The listing builds one solid part. Answer for the finished solid, in the listing's coordinates (mm). Face numbers are marked on the shaded views. A direction names the side the tool comes from. Coordinates: 2 decimals unless noted, no trailing zeros. Write each loop counter-clockwise with the first axis right and the second up, starting at its lowest first coordinate (ties: lowest second). Pieces come first, ordered by that corner, then holes. Notation, with made-up numbers: M -22,-9 L 18,-9 A25 ccw 18,6 Z; hole C -9,20 d5. An arc over 180 degrees is marked long. Put each result on its own line as item: value. Start each with the question number.
```python
from build123d import *

# Parameters (mm, degrees)
F1_DEPTH = 3.68
F2_T     = -1
F3_SIZE2 = 0.5
F3_SIZE  = 1.5
F4_SIZE  = 0.2


with BuildPart() as f1:
    # F0 (on Top) → F1 (new body)
    with BuildSketch(Plane.XY):
        with BuildLine():
            Line((-22.8056685835, -3.0772873983), (-22.8056685835, -6.0772873983))
            ThreePointArc((-22.8056685835, -6.0772873983), (-11.8056685835, 4.9227126017), (-22.8056685835, 15.9227126017))
            Line((-22.8056685835, 15.9227126017), (-22.8056685835, 12.9727126017))
            Line((-22.8056685835, 12.9727126017), (-19.8056685835, 12.9727126017))
            Line((-19.8056685835, 12.9727126017), (-19.8056685835, 9.8727126017))
            Line((-19.8056685835, 9.8727126017), (-22.8056685835, 9.8727126017))
            Line((-22.8056685835, 9.8727126017), (-22.8056685835, 7.1727126017))
            ThreePointArc((-22.8056685835, 7.1727126017), (-20.5556685835, 4.9227126017), (-22.8056685835, 2.6727126017))
            Line((-22.8056685835, 2.6727126017), (-22.8056685835, -0.0772873983))
            Line((-22.8056685835, -0.0772873983), (-25.7056685835, -0.0772873983))
            Line((-25.7056685835, -0.0772873983), (-25.7056685835, -3.0772873983))
            Line((-25.7056685835, -3.0772873983), (-22.8056685835, -3.0772873983))
        make_face()
    extrude(amount=F1_DEPTH)

    # F2
    f2_openings = [f1.faces().sort_by_distance(p)[0] for p in [
        (-18.10535, 4.278135, 3.68),
    ]]
    offset(amount=F2_T, openings=f2_openings, kind=Kind.INTERSECTION)

    # F3
    f3_edges = [f1.edges().sort_by_distance(p)[0] for p in [
        (-20.555669, 4.922713, 3.68),
        (-20.555669, 4.922713, 0),
    ]]
    f3_side = f1.faces().sort_by_distance((-20.555669, 4.922713, 1.84))[0]
    chamfer(f3_edges, length=F3_SIZE, length2=F3_SIZE2, reference=f3_side)

    # F4
    f4_edges = [f1.edges().sort_by_distance(p)[0] for p in [
        (-25.705669, -0.077287, 1.84),
        (-25.705669, -3.077287, 1.84),
        (-22.805669, 9.872713, 1.84),
        (-22.805669, 12.972713, 1.84),
    ]]
    chamfer(f4_edges, length=F4_SIZE)


solid = f1.part
```
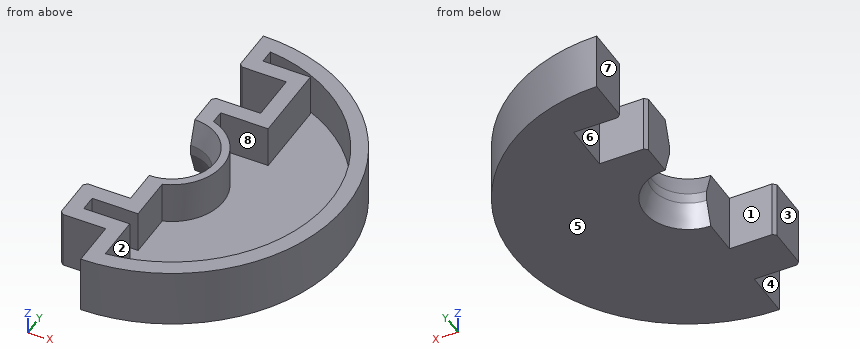
1) A cutting plane is placed at B-B on x = -17.25. Write down the section's boundary in (y, z).
2) Given pin 1 Ø2 at (x, z) = (-19, 2.5) entering from +Y; pin 2 Ø3.5 at (x, y) = (-18, 3) entering from +Z; pin 3 Ø1 at (y, z) = (14.5, 2.5) entering from +X, each flat-ended and moving along its own axis, determine where each tip first touches the part or whether it passes through.
3) A cutting plane is placed at D-D on z = 3.05. Write down the section's boundary in (x, y).
4) For the marked faces 4, 5, 6, 7 and 8, determine the directions among +Z, -Z, +X, -X, +Y, -Y from which every point of the face is accessible in a straight line to the end or side of a thin tool.
5) Determine the mould class of the marked faces 1, 2 and 3 for opening direction Y: +Y half, -Y half, draft (parallel to the pull), parting line (faces both ways), or undercut.
6) A cutting plane is placed at C-C on y = 13.5. Write down the section's boundary in (x, z), then the cut area to 3 significant figures.
7) Straight lines are drawn through the part: probe 1 along Y at (x, z) = (-20.75, 0.7); probe 2 along Y at (x, z) = (-23.75, 2.2); probe 3 along Y at (x, z) = (-21.5, 0.85). For each, find the intervals that lie inside material, in ascending order.
8) A cutting plane is placed at A-A on z = 1.9. Write down the section's boundary in (x, y), then the cut area to 3 significant figures.
Answers follow:
1. outline: M -4.57,0 L 14.42,0 L 14.42,3.68 L 13.24,3.68 L 13.24,1 L -3.39,1 L -3.39,3.68 L -4.57,3.68 Z
2. pin 1: stops at y = 15.56
2. pin 2: stops at z = 1
2. pin 3: stops at x = -16.59
3. outline: M -25.71,-2.88 L -25.51,-3.08 L -22.81,-3.08 L -22.81,-6.08 A11 ccw -22.81,15.92 L -22.81,13.17 L -22.61,12.97 L -19.81,12.97 L -19.81,9.87 L -22.61,9.87 L -22.81,9.67 L -22.81,7.46 A2.54 cw -22.81,2.38 L -22.81,-0.08 L -25.51,-0.08 L -25.71,-0.28 Z; hole M -24.71,-2.08 L -21.81,-2.08 L -21.81,-5.03 A10 ccw -21.81,14.87 L -21.81,13.97 L -18.81,13.97 L -18.81,8.87 L -21.81,8.87 L -21.81,8.02 A3.25 cw -21.81,1.83 L -21.81,-1.08 L -24.71,-1.08 Z
4. face 4: +Z, -Z, -X, -Y
4. face 5: -Z, +X, -X, +Y, -Y
4. face 6: +Z, -Z, -X
4. face 7: +Z, -Z, -X, +Y
4. face 8: +Z
5. face 1: +Y half
5. face 2: undercut
5. face 3: draft
6. outline: M -22.81,0 L -15.92,0 L -15.92,3.68 L -17.66,3.68 L -17.66,1 L -18.81,1 L -18.81,3.68 L -22.81,3.68 Z
6. area: 22.3 mm²
7. probe 1: y = -5.88 to 3.47, 6.37 to 9.87, 12.97 to 15.73
7. probe 2: y = -3.08 to -2.08, -1.08 to -0.08
7. probe 3: y = -6 to 2.83, 7.02 to 9.87, 12.97 to 15.84
8. outline: M -25.71,-2.88 L -25.51,-3.08 L -22.81,-3.08 L -22.81,-6.08 A11 ccw -22.81,15.92 L -22.81,13.17 L -22.61,12.97 L -19.81,12.97 L -19.81,9.87 L -22.61,9.87 L -22.81,9.67 L -22.81,7.17 A2.25 cw -22.81,2.67 L -22.81,-0.08 L -25.51,-0.08 L -25.71,-0.28 Z; hole M -24.71,-2.08 L -21.81,-2.08 L -21.81,-5.03 A10 ccw -21.81,14.87 L -21.81,13.97 L -18.81,13.97 L -18.81,8.87 L -21.81,8.87 L -21.81,8.02 A3.25 cw -21.81,1.83 L -21.81,-1.08 L -24.71,-1.08 Z
8. area: 66.9 mm²
